Check sheet for the modelled part. Datum: model origin and axes. Units: mm. A direction names the side the tool comes from. Round coordinates to 2 decimals unless told otherwise and drop trailing zeros. Loops run counter-clockwise (first coordinate to the right, second up) from the corner with the lowest first, then second, coordinate; pieces in that order, holes last. Notation, with made-up numbers: (39, 31) - (98, 31) arc R18 ccw to (98, 43) - close; hole circle Ø11 at (-17, 13.25). An arc over 180 degrees is marked (long way). Put each result on its own line as item: value.
```python
from build123d import *

# Parameters (mm, degrees)
ESQUISSE1_R             = 13
BOSS_EXTRU_1_DEPTH      = 78.4
ESQUISSE2_R             = 2.5
BOSS_EXTRU_2_DEPTH      = 17
ENL_V_MAT_EXTRU_1_DEPTH = 18.5
ESQUISSE4_R             = 6.5
ESQUISSE4_R_2           = 2.5
BOSS_EXTRU_3_DEPTH      = 2
ESQUISSE5_R             = 1.5
ENL_V_MAT_EXTRU_2_DEPTH = 4
ENL_V_START             = -12
ENL_V_MAT_EXTRU_3_DEPTH = 12


with BuildPart() as part:
    # Esquisse1 → Boss.-Extru.1 (new body)
    with BuildSketch(Plane.XY):
        Circle(ESQUISSE1_R)
    extrude(amount=BOSS_EXTRU_1_DEPTH)

    # Esquisse2 → Boss.-Extru.2 (add)
    with BuildSketch(Plane.XY.offset(78.4)):
        Circle(ESQUISSE2_R)
    extrude(amount=BOSS_EXTRU_2_DEPTH)

    # Esquisse3 → Enlèv. mat.-Extru.1 (cut)
    with BuildSketch(Plane(origin=(0, 0, 0), x_dir=(-1, 0, 0), z_dir=(0, 0, -1))):
        with BuildLine():
            Line((-10.5, 0), (-10.5, 4))
            Line((-10.5, 4), (-12.369316877, 4))
            ThreePointArc((-12.369316877, 4), (-13, 0), (-12.369316877, -4))
            Line((-12.369316877, -4), (-10.5, -4))
            Line((-10.5, -4), (-10.5, 0))
        make_face()
        with BuildLine():
            Line((10.5, 0), (10.5, 4))
            Line((10.5, 4), (12.369316877, 4))
            ThreePointArc((12.369316877, 4), (12.99999812, -0.006990598), (12.365007817, -4.013300596))
            Line((12.365007817, -4.013300596), (10.5, -4))
            Line((10.5, -4), (10.5, 0))
        make_face()
    extrude(amount=-ENL_V_MAT_EXTRU_1_DEPTH, mode=Mode.SUBTRACT)

    # Esquisse4 → Boss.-Extru.3 (add)
    with BuildSketch(Plane.XY.offset(78.4)):
        Circle(ESQUISSE4_R)
        Circle(ESQUISSE4_R_2, mode=Mode.SUBTRACT)
    extrude(amount=BOSS_EXTRU_3_DEPTH)

    # Esquisse5 → Enlèv. mat.-Extru.2 (cut)
    with BuildSketch(Plane.XY.offset(78.4)):
        with Locations((0, 10)):
            Circle(ESQUISSE5_R)
        with Locations((-10, 0)):
            Circle(ESQUISSE5_R)
        with Locations((0, -10)):
            Circle(ESQUISSE5_R)
        with Locations((10, 0)):
            Circle(ESQUISSE5_R)
    extrude(amount=-ENL_V_MAT_EXTRU_2_DEPTH, mode=Mode.SUBTRACT)

    # Esquisse6 → Enlèv. mat.-Extru.3 (cut)
    with BuildSketch(Plane.XY.offset(95.4).offset(ENL_V_START)):
        with BuildLine():
            Line((0, 2), (1.5, 2))
            ThreePointArc((1.5, 2), (0, 2.5), (-1.5, 2))
            Line((-1.5, 2), (0, 2))
        make_face()
    extrude(amount=ENL_V_MAT_EXTRU_3_DEPTH, mode=Mode.SUBTRACT)


solid = part.part
```
Item 1: Section check B-B on z = 7. Enter the section's corners in (x, y) (3 decimals), then the cut area to 3 significant figures.
Filled sheet:
outline: (-12.369, 4) - (-10.5, 4) - (-10.5, -4) - (-12.365, -4.013) arc R13 ccw to (12.369, -4) - (10.5, -4) - (10.5, 4) - (12.369, 4) arc R13 ccw to start
area: 494 mm²
Item 2: Thickness scan on line 1 (Y direction, x = 0, z = 75.95); line 2 (Z direction, x = -1.5, y = 9.25); line 3 (Y direction, x = -0.25, z = 34). Record the ranges inside material, lowest first. Write a range as from..to.
Filled sheet:
line 1: -13..-11.5, -8.5..8.5, 11.5..13
line 2: 0..78.4
line 3: -13..13
Item 3: Section check D-D on y = -5. Enter the section's corners in (x, z).
Filled sheet:
outline: (-12, 0) - (12, 0) - (12, 78.4) - (4.15, 78.4) - (4.15, 80.4) - (-4.15, 80.4) - (-4.15, 78.4) - (-12, 78.4) - close
Item 4: Tool access check on faces 4 (the cylindrical face through (-0.54, -2.44, 87.8)), 5 (the flat face through (-11, 4, 9)), 6 (the flat face through (0, 2, 89)). Record the directions out of +Z, -Z, +X, -X, +Y, -Y that give a thin tool (end or side, any length) a straight path to the whole face; none if there is none.
Filled sheet:
face 4: +Z
face 5: -Z, -X
face 6: +Z, +X, -X, +Y
Item 5: Section check C-C on x = 0. Enter the section's corners in (y, z).
Filled sheet:
outline: (-13, 0) - (13, 0) - (13, 78.4) - (11.5, 78.4) - (11.5, 74.4) - (8.5, 74.4) - (8.5, 78.4) - (6.5, 78.4) - (6.5, 80.4) - (2.5, 80.4) - (2.5, 83.4) - (2, 83.4) - (2, 95.4) - (-2.5, 95.4) - (-2.5, 80.4) - (-6.5, 80.4) - (-6.5, 78.4) - (-8.5, 78.4) - (-8.5, 74.4) - (-11.5, 74.4) - (-11.5, 78.4) - (-13, 78.4) - close
Item 6: Release check for a two-part mould opening along Y. For faces 1 (the flat face through (12, 0, 18.5)), 2 (the flat face through (0, 0, 0)), 3 (the cylindrical face through (-5.158, -3.955, 79.386)) record: +Y half, -Y half, draft (parallel to the pull), parting line (faces both ways), or undercut.
Filled sheet:
face 1: undercut
face 2: draft
face 3: parting line
Item 7: Section check A-A on y = 0. Enter the section's corners in (x, z).
Filled sheet:
outline: (-13, 18.5) - (-10.5, 18.5) - (-10.5, 0) - (10.5, 0) - (10.5, 18.5) - (13, 18.5) - (13, 78.4) - (11.5, 78.4) - (11.5, 74.4) - (8.5, 74.4) - (8.5, 78.4) - (6.5, 78.4) - (6.5, 80.4) - (2.5, 80.4) - (2.5, 95.4) - (-2.5, 95.4) - (-2.5, 80.4) - (-6.5, 80.4) - (-6.5, 78.4) - (-8.5, 78.4) - (-8.5, 74.4) - (-11.5, 74.4) - (-11.5, 78.4) - (-13, 78.4) - close
Item 8: Go/stop test with flat-tipped pins: pin 1 (10 mm diameter, centred on x = 8, y = -2.5, fed in from -Z); pin 2 (0.9 mm diameter, centred on x = -11.5, z = 8, fed in from -Y); pin 3 (5 mm diameter, centred on y = 8.5, z = 67, fed in from -X); pin 4 (1 mm diameter, centred on x = 6.5, y = -6, fed in from +Z). Record where each tip stops, or that it passes through.
Filled sheet:
pin 1: z = 0
pin 2: y = -6.85
pin 3: x = -11.53
pin 4: z = 78.4
